Model file for the job. Use its own axes, mm. Face numbers are marked on the shaded views. Coordinates: 2 decimals unless noted, no trailing zeros. Write each loop counter-clockwise with the first axis right and the second up, starting at its lowest first coordinate (ties: lowest second). Pieces come first, ordered by that corner, then holes. Notation, with made-up numbers: (26, 22.25) - (79, 22.25) arc R20 cw to (79, 50.25) - close; hole circle Ø10 at (73.5, -1.75). An arc over 180 degrees is marked (long way). Put each result on its own line as item: value. Start each with the question number.
1. Saw through at A-A, the plane x = -20. Write the cut outline in (y, z).
2. Pull direction Y, two halves, no side cores. Call the marked faces 1, 2 and 3: released by +Y, released by -Y, zero draft, split by the parting line, or undercut.
3. Saw through at B-B, the plane y = 72.5. Write the cut outline in (x, z).
4. Saw through at D-D, the plane x = -60. Write the cut outline in (y, z).
5. Drop flat-ended pins along their axis: P1, Ø3, axis at x = -65, y = 79, coming from the +Z side; P2, Ø1, axis at x = -58.5, z = 38, coming from the +Y side; P3, Ø12, axis at x = -75, y = 64, coming from the +Z side. Give the stop position or say it passes through.
6. Drill centre lines: L1, parallel to Y at x = -61, z = 10.5; L2, parallel to Y at x = -27, z = 13; L3, parallel to Z at x = 6, y = 38.5. Where is each one in solid material? Low to high. Write a range as from..to.
7. Saw through at C-C, the plane z = 19. Give the number of separate pieces and of enclosed holes in the cut face, plus the area to 3 significant figures.
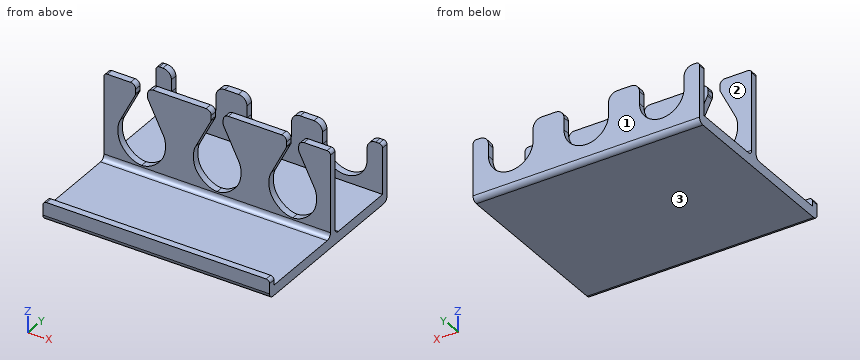
```python
from build123d import *

# Parameters (mm, degrees)
SKETCH1_W           = 238
SKETCH1_H           = 43
SKETCH1_H_2         = 4
SKETCH1_H_3         = 51
BOSS_EXTRUDE1_DEPTH = 6
SKETCH2_W           = 238
SKETCH2_H           = 4
BOSS_EXTRUDE2_DEPTH = 35
SKETCH3_W           = 26
SKETCH3_H           = 12
CUT_EXTRUDE1_DEPTH  = 6
FILLET1_R           = 5
SKETCH4_W           = 238
SKETCH4_H           = 64
BOSS_EXTRUDE3_DEPTH = 4
SKETCH6_W           = 238
SKETCH6_H           = 11
BOSS_EXTRUDE4_DEPTH = 4
CUT_EXTRUDE2_DEPTH  = 10
SKETCH8_W           = 238
SKETCH8_H           = 8
CUT_EXTRUDE3_DEPTH  = 60
FILLET2_R           = 3
FILLET3_R           = 2
FILLET4_R           = 3
CUT_EXTRUDE4_DEPTH  = 150
FILLET5_R           = 2


with BuildPart() as part:
    # Sketch1 → Boss-Extrude1 (new body)
    with BuildSketch(Plane.XY):
        with Locations((0, 54.430088496)):
            Rectangle(SKETCH1_W, SKETCH1_H)
        Polygon((-119, 79.930088496), (-119, 75.930088496), (119, 75.930088496), (119, 79.930088496), (101, 79.930088496), (75, 79.930088496), (57.077876106, 79.930088496), (57, 79.930088496), (31, 79.930088496), (13, 79.930088496), (-13, 79.930088496), (-31, 79.930088496), (-57, 79.930088496), (-75, 79.930088496), (-101, 79.930088496), align=None)
        with Locations((0, 30.930088496)):
            Rectangle(SKETCH1_W, SKETCH1_H_2)
        with Locations((0, 3.430088496)):
            Rectangle(SKETCH1_W, SKETCH1_H_3)
        with Locations((0, -24.069911504)):
            Rectangle(SKETCH1_W, SKETCH1_H_2)
    extrude(amount=BOSS_EXTRUDE1_DEPTH)

    # Sketch2 → Boss-Extrude2 (add)
    with BuildSketch(Plane.XY):
        with Locations((0, 77.930088496)):
            Rectangle(SKETCH2_W, SKETCH2_H)
    extrude(amount=BOSS_EXTRUDE2_DEPTH)

    # Sketch3 → Cut-Extrude1 (cut)
    with BuildSketch(Plane(origin=(0, 79.930088496, 0), x_dir=(1, 0, 0), z_dir=(0, 1, 0))):
        with BuildLine():
            ThreePointArc((-101, -23), (-88, -10), (-75, -23))
            Line((-75, -23), (-101, -23))
        make_face()
        with Locations((-88, -29)):
            Rectangle(SKETCH3_W, SKETCH3_H)
        with BuildLine():
            ThreePointArc((-57, -23), (-44, -10), (-31, -23))
            Line((-31, -23), (-31, -35))
            Line((-31, -35), (-57, -35))
            Line((-57, -35), (-57, -23))
        make_face()
        with BuildLine():
            Line((13, -35), (13, -23))
            ThreePointArc((13, -23), (0, -10), (-13, -23))
            Line((-13, -23), (-13, -35))
            Line((-13, -35), (13, -35))
        make_face()
        with BuildLine():
            Line((57, -35), (57, -23))
            ThreePointArc((57, -23), (44, -10), (31, -23))
            Line((31, -23), (31, -35))
            Line((31, -35), (57, -35))
        make_face()
        with BuildLine():
            Line((101, -35), (101, -23))
            ThreePointArc((101, -23), (88, -10), (75, -23))
            Line((75, -23), (75, -35))
            Line((75, -35), (101, -35))
        make_face()
    extrude(amount=-CUT_EXTRUDE1_DEPTH, mode=Mode.SUBTRACT)

    # Fillet1
    fillet1_edges = [part.edges().sort_by_distance(p)[0] for p in [
        (-119, 77.930088496, 35),
        (119, 77.930088496, 35),
        (75, 77.930088496, 35),
        (101, 77.930088496, 35),
        (31, 77.930088496, 35),
        (57, 77.930088496, 35),
        (-13, 77.930088496, 35),
        (13, 77.930088496, 35),
        (-57, 77.930088496, 35),
        (-31, 77.930088496, 35),
        (-101, 77.930088496, 35),
        (-75, 77.930088496, 35),
    ]]
    fillet(fillet1_edges, radius=FILLET1_R)

    # Sketch4 → Boss-Extrude3 (add)
    with BuildSketch(Plane(origin=(0, 32.930088496, 0), x_dir=(1, 0, 0), z_dir=(0, 1, 0))):
        with Locations((0, -32)):
            Rectangle(SKETCH4_W, SKETCH4_H)
    extrude(amount=-BOSS_EXTRUDE3_DEPTH)

    # Sketch6 → Boss-Extrude4 (add)
    with BuildSketch(Plane(origin=(0, -22.069911504, 0), x_dir=(1, 0, 0), z_dir=(0, 1, 0))):
        with Locations((0, -5.5)):
            Rectangle(SKETCH6_W, SKETCH6_H)
    extrude(amount=-BOSS_EXTRUDE4_DEPTH)

    # Sketch5 → Cut-Extrude2 (cut)
    with BuildSketch(Plane(origin=(0, 32.930088496, 0), x_dir=(1, 0, 0), z_dir=(0, 1, 0))):
        with BuildLine():
            Line((-40.5, -50), (-40.5, -56))
            Line((-40.5, -56), (-47.5, -56))
            Line((-47.5, -56), (-47.5, -50))
            Line((-47.5, -50), (-56.5, -32))
            add(Edge.make_bspline(
                [(-56.5, -32), (-58.118524022, -29.356350797), (-58.608084098, -22.1569248), (-53.268932872, -13.423946955), (-48.161141466, -10.022473266), (-44, -10)],
                knots=[0, 0, 0, 0, 0.224491173, 0.274489259, 0.499980858, 0.499980858, 0.499980858, 0.499980858], degree=3))
            add(Edge.make_bspline(
                [(-31.5, -32), (-29.881475978, -29.356350797), (-29.391915902, -22.1569248), (-34.731067128, -13.423946955), (-39.838858534, -10.022473266), (-44, -10)],
                knots=[0, 0, 0, 0, 0.224491173, 0.274489259, 0.499980858, 0.499980858, 0.499980858, 0.499980858], degree=3))
            Line((-31.5, -32), (-40.5, -50))
        make_face()
        with BuildLine():
            Line((-84.5, -50), (-75.5, -32))
            add(Edge.make_bspline(
                [(-75.5, -32), (-73.881475978, -29.356350797), (-73.391915902, -22.1569248), (-78.731067128, -13.423946955), (-83.838858534, -10.022473266), (-88, -10)],
                knots=[0, 0, 0, 0, 0.224491173, 0.274489259, 0.499980858, 0.499980858, 0.499980858, 0.499980858], degree=3))
            add(Edge.make_bspline(
                [(-100.5, -32), (-102.118524022, -29.356350797), (-102.608084098, -22.1569248), (-97.268932872, -13.423946955), (-92.161141466, -10.022473266), (-88, -10)],
                knots=[0, 0, 0, 0, 0.224491173, 0.274489259, 0.499980858, 0.499980858, 0.499980858, 0.499980858], degree=3))
            Line((-100.5, -32), (-91.5, -50))
            Line((-91.5, -50), (-91.5, -56))
            Line((-91.5, -56), (-84.5, -56))
            Line((-84.5, -56), (-84.5, -50))
        make_face()
        with BuildLine():
            Line((3.5, -50), (12.5, -32))
            add(Edge.make_bspline(
                [(12.5, -32), (14.118524022, -29.356350797), (14.608084098, -22.1569248), (9.268932872, -13.423946955), (4.161141466, -10.022473266), (0, -10)],
                knots=[0, 0, 0, 0, 0.224491173, 0.274489259, 0.499980858, 0.499980858, 0.499980858, 0.499980858], degree=3))
            add(Edge.make_bspline(
                [(-12.5, -32), (-14.118524022, -29.356350797), (-14.608084098, -22.1569248), (-9.268932872, -13.423946955), (-4.161141466, -10.022473266), (0, -10)],
                knots=[0, 0, 0, 0, 0.224491173, 0.274489259, 0.499980858, 0.499980858, 0.499980858, 0.499980858], degree=3))
            Line((-12.5, -32), (-3.5, -50))
            Line((-3.5, -50), (-3.5, -56))
            Line((-3.5, -56), (3.5, -56))
            Line((3.5, -56), (3.5, -50))
        make_face()
    extrude(amount=-CUT_EXTRUDE2_DEPTH, mode=Mode.SUBTRACT)

    # Sketch8 → Cut-Extrude3 (cut)
    with BuildSketch(Plane(origin=(0, 0, 0), x_dir=(1, 0, 0), z_dir=(0, 1, 0))):
        with Locations((0, -60)):
            Rectangle(SKETCH8_W, SKETCH8_H)
    extrude(amount=CUT_EXTRUDE3_DEPTH, mode=Mode.SUBTRACT)

    # Fillet2
    fillet2_edges = [part.edges().sort_by_distance(p)[0] for p in [
        (-84.5, 30.930088496, 56),
        (-91.5, 30.930088496, 56),
        (3.5, 30.930088496, 56),
        (-3.5, 30.930088496, 56),
        (-40.5, 30.930088496, 56),
        (-47.5, 30.930088496, 56),
    ]]
    fillet(fillet2_edges, radius=FILLET2_R)

    # Fillet3
    fillet3_edges = [part.edges().sort_by_distance(p)[0] for p in [
        (-84.5, 30.930088496, 50),
        (-91.5, 30.930088496, 50),
        (3.5, 30.930088496, 50),
        (-3.5, 30.930088496, 50),
        (-40.5, 30.930088496, 50),
        (-47.5, 30.930088496, 50),
    ]]
    fillet(fillet3_edges, radius=FILLET3_R)

    # Fillet4
    fillet4_edges = [part.edges().sort_by_distance(p)[0] for p in [
        (0, 28.930088496, 6),
        (0, 32.930088496, 6),
        (0, -26.069911504, 0),
        (0, 79.930088496, 0),
    ]]
    fillet(fillet4_edges, radius=FILLET4_R)

    # Sketch9 → Cut-Extrude4 (cut, symmetric)
    with BuildSketch(Plane(origin=(0, 0, 0), x_dir=(1, 0, 0), z_dir=(0, 1, 0))):
        Polygon((-110, -70.570691383), (-110, -35), (-110, 17.336036992), (-146.355677451, 17.336036992), (-144.312296295, -70.570691383), align=None)
        Polygon((136.221626858, 30.554600482), (22, 30.554600482), (22, -35), (22, -79.242199879), (136.221626858, -79.242199879), align=None)
    extrude(amount=CUT_EXTRUDE4_DEPTH, both=True, mode=Mode.SUBTRACT)

    # Fillet5
    fillet5_edges = [part.edges().sort_by_distance(p)[0] for p in [
        (-110, 77.930088496, 35),
        (-110, 30.930088496, 56),
        (-110, -24.069911504, 11),
        (22, 30.930088496, 56),
        (22, -24.069911504, 11),
        (22, 77.930088496, 35),
    ]]
    fillet(fillet5_edges, radius=FILLET5_R)


solid = part.part
```
Final values:
1. outline: (-26.07, 3) arc R3 ccw to (-23.07, 0) - (76.93, 0) arc R3 ccw to (79.93, 3) - (79.93, 35) - (75.93, 35) - (75.93, 6) - (35.93, 6) arc R3 cw to (32.93, 9) - (32.93, 56) - (28.93, 56) - (28.93, 9) arc R3 cw to (25.93, 6) - (-22.07, 6) - (-22.07, 11) - (-26.07, 11) - close
2. face 1: released by +Y
2. face 2: undercut
2. face 3: zero draft
3. outline: (-110, 0) - (22, 0) - (22, 6) - (-110, 6) - close
4. outline: (-26.07, 3) arc R3 ccw to (-23.07, 0) - (76.93, 0) arc R3 ccw to (79.93, 3) - (79.93, 34.58) - (75.93, 34.58) - (75.93, 6) - (35.93, 6) arc R3 cw to (32.93, 9) - (32.93, 56) - (28.93, 56) - (28.93, 9) arc R3 cw to (25.93, 6) - (-22.07, 6) - (-22.07, 11) - (-26.07, 11) - close
5. P1: stops at z = 35
5. P2: stops at y = 32.93
5. P3: stops at z = 6
6. L1: y = -26.07..-22.07, 28.93..32.93, 75.93..79.93
6. L2: y = 28.93..32.93, 75.93..79.93
6. L3: z = 0..6
7. separate pieces: 8
7. enclosed holes: 0
7. area: 458 mm²
